from build123d import *

# Parameters (mm, degrees)
F0_W      = 145
F0_H      = 5
F1_DEPTH  = 360
F0_W_2    = 58
F0_H_2    = 655
F2_DEPTH  = 360
F0_W_3    = 155
F0_H_3    = 163
F0_H_4    = 153
F3_DEPTH  = 360
F5_DEPTH  = 665
F7_DEPTH  = 394
F9_DEPTH  = 125
F11_DEPTH = 50
F12_R     = 5
F14_R     = 2.5
F15_DEPTH = 10
F13_R     = 2.5
F16_DEPTH = 10
F18_DEPTH = 502


# Not quite as in the source:
# - a feature names something its author has since deleted; it is built from what else it names


with BuildPart() as f1:
    # F0 (on Top) → F1 (new body)
    with BuildSketch(Plane.XY):
        Polygon((5, 0), (0, 0), (0, -665), (5, -665), (5, -660), (5, -5), align=None)
        Polygon((155, 0), (5, 0), (5, -5), (150, -5), (155, -5), align=None)
        Polygon((155, -665), (155, -5), (150, -5), (150, -660), (150, -665), align=None)
        with Locations((77.5, -662.5)):
            Rectangle(F0_W, F0_H)
    extrude(amount=-F1_DEPTH)


with BuildPart() as f2:
    # F0 (on Top) → F2 (new body)
    with BuildSketch(Plane.XY):
        Polygon((239, 0), (155, 0), (155, -5), (155, -665), (239, -665), (239, -163), align=None)
        with Locations((197, -332.5)):
            Rectangle(F0_W_2, F0_H_2, mode=Mode.SUBTRACT)
    extrude(amount=-F2_DEPTH)


with BuildPart() as f3:
    # F0 (on Top) → F3 (new body)
    with BuildSketch(Plane.XY):
        with Locations((316.5, -81.5)):
            Rectangle(F0_W_3, F0_H_3)
        with Locations((316.5, -81.5)):
            Rectangle(F0_W, F0_H_4, mode=Mode.SUBTRACT)
    extrude(amount=-F3_DEPTH)


with BuildPart() as f5:
    # F4 (on face) → F5 (new body)
    with BuildSketch(Plane(origin=(0, 0, 0), x_dir=(-1, 0, 0), z_dir=(0, 1, 0))):
        Polygon((0, -330), (0, -360), (30, -360), (30, -359), (1, -359), (1, -330), align=None)
    extrude(amount=-F5_DEPTH)


with BuildPart() as f7:
    # F6 (on face) → F7 (new body)
    with BuildSketch(Plane.YZ.offset(394)):
        Polygon((0, -330), (0, -360), (30, -360), (30, -359), (1, -359), (1, -330), align=None)
    extrude(amount=-F7_DEPTH)


with BuildPart() as f9:
    # F8 (on face) → F9 (new body)
    with BuildSketch(Plane.YZ.offset(394)):
        Polygon((-193, -360), (-163, -360), (-163, -330), (-164, -330), (-164, -359), (-193, -359), align=None)
    extrude(amount=-F9_DEPTH)


with BuildPart() as f11:
    # F10 (on face) → F11 (new body)
    with BuildSketch(Plane.YZ.offset(239)):
        Polygon((-698, -360), (-665, -360), (-665, -327), (-668, -327), (-668, -357), (-698, -357), align=None)
    extrude(amount=-F11_DEPTH)

    # F12
    f12_edges = [f11.edges().sort_by_distance(p)[0] for p in [
        (214, -668, -357),
        (189, -666.5, -327),
        (239, -666.5, -327),
        (239, -698, -358.5),
        (189, -698, -358.5),
        (214, -665, -360),
    ]]
    fillet(f12_edges, radius=F12_R)


with BuildPart() as f15_tool:
    # F14 (on face) → F15 (new body)
    with BuildSketch(Plane.XZ.offset(668)):
        with Locations((204, -342)):
            Circle(F14_R)
        with Locations((224, -342)):
            Circle(F14_R)
    extrude(amount=-F15_DEPTH)


with BuildPart() as f2_1:
    add(f2.part)

    # F15: cut by f15_tool
    add(f15_tool.part, mode=Mode.SUBTRACT)


with BuildPart() as f11_1:
    add(f11.part)

    # F15: cut by f15_tool
    add(f15_tool.part, mode=Mode.SUBTRACT)

    # F13 (on face) → F16 (cut)
    with BuildSketch(Plane.XY.offset(-357)):
        with Locations((204, -683)):
            Circle(F13_R)
        with Locations((224, -683)):
            Circle(F13_R)
    extrude(amount=-F16_DEPTH, mode=Mode.SUBTRACT)


with BuildPart() as f18:
    # F17 (on face) → F18 (new body)
    with BuildSketch(Plane.XZ.offset(665)):
        Polygon((242, -330), (239, -330), (239, -360), (269, -360), (269, -357), (242, -357), align=None)
    extrude(amount=-F18_DEPTH)


solid = f11_1.part
Model file for the job. Use its own axes, mm. A direction names the side the tool comes from. Give positions to 0.01 mm unless a question says otherwise; leave off trailing zeros. Order: outer loops, then holes, each group sorted by start corner. A loop starts at its lowest first (then second) coordinate and runs counter-clockwise, first axis right, second up. Notation, with made-up numbers: M -23.5,50 L -7.5,50 A21 cw -7.5,66 Z; hole C -31.75,-36.5 d10. An arc over 180 degrees is marked long. Write item = value, one per line.
Q1. Two-plate mould, pull along Y, no slides. Class faces 1 (the cylindrical face through (205.15, -666.52, -344.22)), 2 (the cylindrical face through (214, -667, -359)), 3 (the cylindrical face through (205.34, -680.89, -358.48)), 4 (the cylindrical face through (225.34, -680.89, -358.48)): pulls with the +Y half, pulls with the -Y half, needs draft (parallel to the pull), parting line crosses it, or undercut.
Derived:
face_1 = needs draft
face_2 = pulls with the +Y half
face_3 = undercut
face_4 = undercut
Q2. Drill centre lines: line 1 (X direction, y = -666.8, z = -342); line 2 (Y direction, x = 193.5, z = -337.5); line 3 (Y direction, x = 224, z = -358). Where is each one in solid material? Low to high. Write a range as [from, to].
Derived:
line_1 = [189, 201.5], [206.5, 221.5], [226.5, 239]
line_2 = [-668, -665]
line_3 = [-698, -685.5], [-680.5, -666]
Q3. Cut at D-D, the plane z = -337. List the corners of the cut face in (x, y).
Derived:
outline = M 189,-668 L 239,-668 L 239,-665 L 189,-665 Z
Q4. Tool access for faces 5 (the cylindrical face through (191, -697, -359)), 6 (the flat face through (214, -668, -339)): list every direction of +Z, -Z, +X, -X, +Y, -Y with a clear straight run to the whole face (end or side of a thin tool).
Derived:
face_5 = +Z, -Z, -X, -Y
face_6 = +Z, +X, -X, -Y
Q5. Cut at A-A, the plane z = -342. List the corners of the cut face in (x, y), then the cut area to 3 significant figures.
Derived:
outline = M 189,-668 L 201.5,-668 L 201.5,-665 L 189,-665 Z; M 206.5,-668 L 221.5,-668 L 221.5,-665 L 206.5,-665 Z; M 226.5,-668 L 239,-668 L 239,-665 L 226.5,-665 Z
area = 120 mm2
Q6. Cut at C-C, the plane x = 217. List the corners of the cut face in (y, z).
Derived:
outline = M -698,-360 L -670,-360 A5 ccw -665,-355 L -665,-327 L -668,-327 L -668,-352 A5 cw -673,-357 L -698,-357 Z
Q7. Flat gauge pins, fed straight in: pin 1 (4 mm diameter, centred on x = 204, y = -683, fed in from -Z); pin 2 (4 mm diameter, centred on x = 202, z = -344, fed in from -Y); pin 3 (6 mm diameter, centred on x = 206.5, y = -683, fed in from +Z). Where does each tip first touch, or does it go through?
Derived:
pin_1 = through
pin_2 = -668
pin_3 = -357
Q8. Cut at B-B, the plane x = 224. List the corners of the cut face in (y, z).
Derived:
outline = M -698,-360 L -685.5,-360 L -685.5,-357 L -698,-357 Z; M -680.5,-360 L -670,-360 A5 ccw -665,-355 L -665,-344.5 L -668,-344.5 L -668,-352 A5 cw -673,-357 L -680.5,-357 Z; M -668,-339.5 L -665,-339.5 L -665,-327 L -668,-327 Z
